Source: CAD feature listing. Evaluate the final solid. Frame: model axes, mm. Face numbers are marked on the shaded views. A direction names the side the tool comes from. Coordinates: 2 decimals unless noted, no trailing zeros. Write each loop counter-clockwise with the first axis right and the second up, starting at its lowest first coordinate (ties: lowest second). Pieces come first, ordered by that corner, then holes. Notation, with made-up numbers: (-30, 34.25) - (0, 34.25) arc R27 ccw to (0, 69.25) - close; hole circle Ø6 at (36.25, 71). An arc over 180 degrees is marked (long way). One line per question, with ' | ' between items.
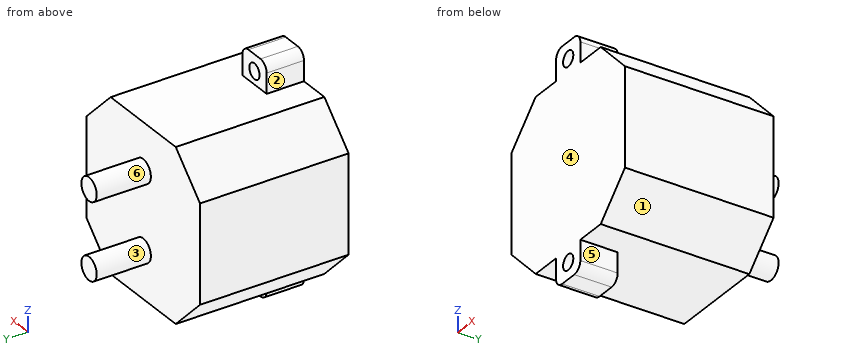
from build123d import *

# Parameters (mm, degrees)
BOSS_EXTRUDE1_DEPTH = 12.954
BOSS_EXTRUDE2_DEPTH = 38.608
SKETCH3_R           = 2.667
CUT_EXTRUDE1_DEPTH  = 100.331862844
FILLET1_R           = 3.175
SKETCH4_R           = 4
BOSS_EXTRUDE3_DEPTH = 18.796


with BuildPart() as part:
    # Sketch1 → Boss-Extrude1 (new body)
    with BuildSketch(Plane(origin=(0, 0, 0), x_dir=(1, 0, 0), z_dir=(0, 1, 0))):
        Polygon((36.068, 0), (29.718, 0), (23.368, 0), (23.368, -10.16), (36.068, -10.16), align=None)
        Polygon((36.068, 59.436), (29.718, 59.436), (29.718, 0), (36.068, 0), (46.736, 0), (59.436, 12.7), (59.436, 46.736), (46.736, 59.436), align=None)
        Polygon((29.718, 0), (29.718, 59.436), (23.368, 59.436), (12.7, 59.436), (0, 46.736), (0, 12.7), (12.7, 0), (23.368, 0), align=None)
        Polygon((23.368, 59.436), (29.718, 59.436), (36.068, 59.436), (36.068, 69.596), (23.368, 69.596), align=None)
    extrude(amount=BOSS_EXTRUDE1_DEPTH)

    # Sketch2 → Boss-Extrude2 (add)
    with BuildSketch(Plane(origin=(0, 12.954, 0), x_dir=(1, 0, 0), z_dir=(0, 1, 0))):
        Polygon((23.368, 59.436), (36.068, 59.436), (46.736, 59.436), (59.436, 46.736), (59.436, 12.7), (46.736, 0), (36.068, 0), (23.368, 0), (12.7, 0), (0, 12.7), (0, 46.736), (12.7, 59.436), align=None)
    extrude(amount=BOSS_EXTRUDE2_DEPTH)

    # Sketch3 → Cut-Extrude1 (cut, through all)
    with BuildSketch(Plane(origin=(0, 12.954, 0), x_dir=(1, 0, 0), z_dir=(0, 1, 0))):
        with Locations(Location((29.718, 63.881, 0), (0, 0, 270))):
            Circle(SKETCH3_R)
        with Locations(Location((29.718, -4.445, 0), (0, 0, 270))):
            Circle(SKETCH3_R)
    extrude(amount=-CUT_EXTRUDE1_DEPTH, mode=Mode.SUBTRACT)

    # Fillet1
    fillet1_edges = [part.edges().sort_by_distance(p)[0] for p in [
        (36.068, 6.477, 10.16),
        (23.368, 6.477, 10.16),
        (23.368, 6.477, -69.596),
        (36.068, 6.477, -69.596),
    ]]
    fillet(fillet1_edges, radius=FILLET1_R)

    # Sketch4 → Boss-Extrude3 (add)
    with BuildSketch(Plane(origin=(0, 51.562, 0), x_dir=(1, 0, 0), z_dir=(0, 1, 0))):
        with Locations(Location((29.718, 43.053, 0), (0, 0, 270))):
            Circle(SKETCH4_R)
        with Locations(Location((29.718, 16.383, 0), (0, 0, 270))):
            Circle(SKETCH4_R)
    extrude(amount=BOSS_EXTRUDE3_DEPTH)


solid = part.part
Item 1: Cut plane B-B on z = 5. Return loops of the section in (x, y), and give its area (3 significant figures).
Check sheet entries:
outline: (23.37, 0) - (27.11, 0) - (27.11, 12.95) - (23.37, 12.95) - close; (32.33, 0) - (36.07, 0) - (36.07, 12.95) - (32.33, 12.95) - close | area: 96.9 mm²
Item 2: Mould query, pull axis Z, two halves, no side actions, for the marked faces 1, 2 and 3. Classes: pulls with the +Z half, pulls with the -Z half, needs draft (parallel to the pull), parting line crosses it, or undercut.
Check sheet entries:
face 1: pulls with the -Z half | face 2: needs draft | face 3: undercut
Item 3: Cut plane A-A on y = 35. Return loops of the section in (x, z), and give its area (3 significant figures).
Check sheet entries:
outline: (0, -46.74) - (12.7, -59.44) - (46.74, -59.44) - (59.44, -46.74) - (59.44, -12.7) - (46.74, 0) - (12.7, 0) - (0, -12.7) - close | area: 3,210 mm²
Item 4: Pin query (flat end, axial travel): pin 1 Ø4 at (y, z) = (50.5, -6.5) entering from -X; pin 2 Ø17 at (x, y) = (30, 36) entering from +Z; pin 3 Ø3 at (x, z) = (28.5, -62.5) entering from +Y; pin 4 Ø6 at (x, z) = (30.5, -38) entering from +Y. Return the tip coordinate at first contact, or that it passes through.
Check sheet entries:
pin 1: x = 4.2 | pin 2: z = 0 | pin 3: y = 12.95 | pin 4: y = 70.36
Item 5: Cut plane C-C on x = 38. Return loops of the section in (y, z).
Check sheet entries:
outline: (0, -59.44) - (51.56, -59.44) - (51.56, 0) - (0, 0) - close
Item 6: Cut plane D-D on z = -14.5. Return loops of the section in (x, y).
Check sheet entries:
outline: (0, 0) - (59.44, 0) - (59.44, 51.56) - (33.25, 51.56) - (33.25, 70.36) - (26.19, 70.36) - (26.19, 51.56) - (0, 51.56) - close
Item 7: Ray query, line 1 along Z through (x, y) = (31, 12); line 2 along Z through (x, y) = (33, 48.5); line 3 along Y through (x, z) = (15.5, -4.5). Return the intervals inside material, ascending. Write a range as [from, to].
Check sheet entries:
line 1: [-69.6, -66.22], [-61.54, 2.11], [6.78, 10.16] | line 2: [-59.44, 0] | line 3: [0, 51.56]
Item 8: Access query for the marked faces 4, 5 and 6. Directions: +Z, -Z, +X, -X, +Y, -Y. A direction counts if a zero-diameter tool reaches every point of the face in a straight line with its end or side. Return the directions, or none.
Check sheet entries:
face 4: +Z, -Z, +X, -X, -Y | face 5: -Z, +X, +Y, -Y | face 6: +Y
